from build123d import *

# Parameters (mm, degrees)
BOX002_W     = 1
BOX002_H     = 9
BOX002_DEPTH = 9
BOX003_W     = 12
BOX003_H     = 1
BOX003_DEPTH = 9
BOX004_W     = 1
BOX004_H     = 3
BOX004_DEPTH = 3
BOX099_W     = 1
BOX099_H     = 8
BOX099_DEPTH = 9


with BuildPart() as box002:
    # Box002 → Box002 (new body)
    with BuildSketch(Plane(origin=(16, 15, 1), x_dir=(1, 0, 0), z_dir=(0, 0, 1))):
        with Locations((0.5, 4.5)):
            Rectangle(BOX002_W, BOX002_H)
    extrude(amount=BOX002_DEPTH)


with BuildPart() as box003:
    # Box003 → Box003 (new body)
    with BuildSketch(Plane(origin=(1, 15, 1), x_dir=(1, 0, 0), z_dir=(0, 0, 1))):
        with Locations((6, 0.5)):
            Rectangle(BOX003_W, BOX003_H)
    extrude(amount=BOX003_DEPTH)


with BuildPart() as fusion030:
    # Box004 → Box004 (new body)
    with BuildSketch(Plane(origin=(16, 15, 7), x_dir=(0, 1, 0), z_dir=(0, 0, 1))):
        with Locations((0.5, 1.5)):
            Rectangle(BOX004_W, BOX004_H)
    extrude(amount=BOX004_DEPTH)

    # Fusion030: union Box002, Box003
    add(box002.part)
    add(box003.part)


with BuildPart() as fusion030_1:
    # Fusion030 placement: moved
    add(fusion030.part.moved(Location((9, 0, 0))))


with BuildPart() as fusion039:
    # Box099 → Box099 (new body)
    with BuildSketch(Plane(origin=(10, 16, 1), x_dir=(1, 0, 0), z_dir=(0, 0, 1))):
        with Locations((0.5, 4)):
            Rectangle(BOX099_W, BOX099_H)
    extrude(amount=BOX099_DEPTH)

    # Fusion039: union Fusion030
    add(fusion030_1.part)


solid = fusion039.part
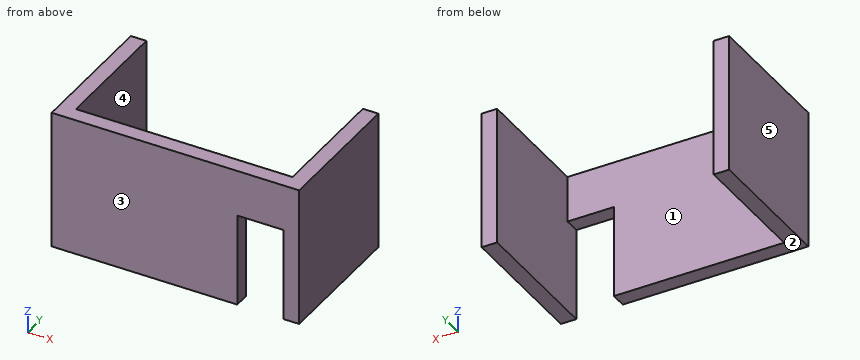
Geometry: final body of the model. Coordinates: model frame, mm. Face numbers are marked on the shaded views. A direction names the side the tool comes from. Round coordinates to 2 decimals unless told otherwise and drop trailing zeros. Loops run counter-clockwise (first coordinate to the right, second up) from the corner with the lowest first, then second, coordinate; pieces in that order, holes last. Notation, with made-up numbers: (80, 66.25) -> (122, 66.25) arc R14 cw to (122, 91.25) -> close; hole circle Ø10 at (25.5, -37.75). An arc over 180 degrees is marked (long way). One line per question, with ' | ' between items. Start each with the question number.
1. Section D-D on y = 15.5. Output: boundary loops of the cut face in (x, z).
2. Set-up query: the marked faces 1 and 2. Return all of +Z, -Z, +X, -X, +Y, -Y with unobstructed straight access to the full face (end or side cutting, diameter ignored); none if empty.
3. Line query: line 1 along X through (y, z) = (17.75, 6.75); line 2 along Y through (x, z) = (14.5, 2.75); line 3 along X through (y, z) = (15.5, 1.5). Output: solid intervals per line, ascending. Write a range as [from, to].
4. Section A-A on y = 16.75. Output: boundary loops of the cut face in (x, z), and give its area (3 significant figures).
5. Mould query, pull axis X, two halves, no side actions, for the marked faces 3, 4 and 5. Classes: pulls with the +X half, pulls with the -X half, needs draft (parallel to the pull), parting line crosses it, or undercut.
6. Section C-C on z = 8.5. Output: boundary loops of the cut face in (x, y).
7. Section B-B on z = 3. Output: boundary loops of the cut face in (x, y), and give its area (3 significant figures).
8. Contact query for flat-ended pins moving along their axis: pin 1 (4.5 mm diameter, centred on x = 20, z = 4, fed in from +Y); pin 2 (1.1 mm diameter, centred on x = 24, y = 15.5, fed in from -Z). Output: stop coordinate, or through.
Returned:
1) outline: (10, 1) -> (22, 1) -> (22, 7) -> (25, 7) -> (25, 1) -> (26, 1) -> (26, 10) -> (10, 10) -> close
2) face 1: +Z, -Z, +Y | face 2: -Z, +X, -X, +Y, -Y
3) line 1: x = [10, 11], [25, 26] | line 2: y = [15, 16] | line 3: x = [10, 22], [25, 26]
4) outline: (10, 1) -> (11, 1) -> (11, 10) -> (10, 10) -> close; (25, 1) -> (26, 1) -> (26, 10) -> (25, 10) -> close | area: 18.0 mm2
5) face 3: needs draft | face 4: undercut | face 5: pulls with the -X half
6) outline: (10, 15) -> (26, 15) -> (26, 24) -> (25, 24) -> (25, 16) -> (11, 16) -> (11, 24) -> (10, 24) -> close
7) outline: (10, 15) -> (22, 15) -> (22, 16) -> (11, 16) -> (11, 24) -> (10, 24) -> close; (25, 15) -> (26, 15) -> (26, 24) -> (25, 24) -> close | area: 29.0 mm2
8) pin 1: stops at y = 16 | pin 2: stops at z = 7
